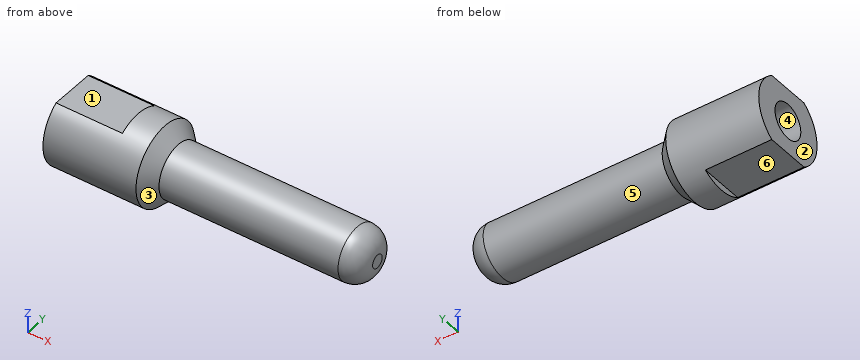
from build123d import *

# Parameters (mm, degrees)
F0_W        = 15.4432
F0_H        = 9.525
F3_DEPTH    = 15.875
F4_R        = 4.7752
F5_S5_R     = 6.35
F5_T6_DEPTH = 15
F7_D        = 8.4328
F7_DEPTH    = 19.685
F7_TIP      = 2.5334687141


# Not quite as in the source:
# - a fillet or chamfer that OpenCascade refuses, or shapes differently, is made with other operations: its cross-section is extruded or revolved along the edge and cut away or added


with BuildPart() as f1:
    # F0 (on Top) → F1 (revolve)
    with BuildSketch(Plane.XY):
        with Locations((-16.8899756006, 4.7625)):
            Rectangle(F0_W, F0_H)
        Polygon((-9.1683756006, 9.525), (-9.1683756006, 0), (48.4134243994, 0), (48.4134243994, 6.35), (0.8138243994, 6.35), (0.8138243994, 9.525), align=None)
    revolve(axis=Axis((11.9009243994, 0, 0), (1, 0, 0)))

    # F2 (on face) → F3 (cut)
    with BuildSketch(Plane(origin=(-24.6115756006, 0, 0), x_dir=(0, -1, 0), z_dir=(-1, 0, 0))):
        with BuildLine():
            ThreePointArc((5.2459455735, 7.9502), (0, 9.525), (-5.2459455735, 7.9502))
            Line((-5.2459455735, 7.9502), (5.2459455735, 7.9502))
        make_face()
        with BuildLine():
            Line((5.2651418547, -7.9375), (-5.2651418547, -7.9375))
            ThreePointArc((-5.2651418547, -7.9375), (0, -9.525), (5.2651418547, -7.9375))
        make_face()
    extrude(amount=-F3_DEPTH, mode=Mode.SUBTRACT)

    # F4
    f4_edges = [f1.edges().sort_by_distance(p)[0] for p in [
        (48.413424, -6.35, 0),
    ]]
    fillet(f4_edges, radius=F4_R)

    # F5: chamfer of 3.175 on 1 edges, made by hand


with BuildPart() as f5_tool2:
    # F5_s3 → F5_t4 (revolve)
    with BuildSketch(Plane.XY):
        Polygon((0.8138243994, 6.35), (-2.3611756006, 9.525), (0.8138243994, 9.525), align=None)
    revolve(axis=Axis((0.8138243994, 0, 0), (1, 0, 0)))

    # F5_s5 → F5_t6 (cut, symmetric)
    with BuildSketch(Plane.YZ.offset(-0.8)):
        Circle(F5_S5_R)
    extrude(amount=F5_T6_DEPTH, both=True, mode=Mode.SUBTRACT)


with BuildPart() as f1_1:
    add(f1.part)

    # F5_t1: cut F5_tool2
    add(f5_tool2.part, mode=Mode.SUBTRACT)

    # F7
    with Locations(Plane(origin=(-24.6115756006, 0, 0), x_dir=(0, -1, 0), z_dir=(-1, 0, 0))):
        with Locations((0, 0)):
            Hole(F7_D / 2, depth=F7_DEPTH)
            with Locations((0, 0, -(F7_DEPTH + F7_TIP / 2))):  # 118° drill point
                Cone(0, F7_D / 2, F7_TIP, mode=Mode.SUBTRACT)


solid = f1_1.part
Model file for the job. Use its own axes, mm. Face numbers are marked on the shaded views. A direction names the side the tool comes from. Round coordinates to 2 decimals unless told otherwise and drop trailing zeros. Loops run counter-clockwise (first coordinate to the right, second up) from the corner with the lowest first, then second, coordinate; pieces in that order, holes last. Notation, with made-up numbers: (8.25, 45.25) - (46.25, 45.25) arc R9 cw to (46.25, 54.25) - close; hole circle Ø9 at (27.5, 53.25). An arc over 180 degrees is marked (long way). Write each question's results on one line, items separated by ' | '.
(1) Pin check, flat tips, straight feed: pin 1 (4 mm diameter, centred on x = -8.5, z = -2.5, fed in from -Y); pin 2 (7.5 mm diameter, centred on y = 0, z = 0, fed in from -X); pin 3 (1.3 mm diameter, centred on y = 1.5, z = 8.5, fed in from -X); pin 4 (3 mm diameter, centred on x = -18.5, y = 1.5, fed in from -Z). Stop position of each tip, or through.
Answer below:
pin 1: stops at y = -9.51 | pin 2: stops at x = -4.65 | pin 3: stops at x = -24.61 | pin 4: stops at z = -7.94
(2) Mould opens along X. For the marked faces 1, 2 and 3 say: released by +X, released by -X, zero draft, split by the parting line, or undercut.
Answer below:
face 1: zero draft | face 2: released by -X | face 3: released by +X
(3) 3-axis set-ups, long thin cutter, end or side, ignore diameter. For the marked faces 4, 5 and 6: which of +Z, -Z, +X, -X, +Y, -Y reach the whole face in a straight line?
Answer below:
face 4: -X | face 5: +X | face 6: -Z, -X, +Y, -Y
(4) Saw through at A-A, the plane x = 33.5. List the corners of the cut face in (y, z), then the cut area to 3 significant figures.
Answer below:
outline: circle Ø12.7 at (0, 0) | area: 127 mm^2
(5) Wall check: L1, parallel to Z at x = -18.75, y = 0; L2, parallel to Y at x = -19.25, z = 0 (3 decimals); L3, parallel to Y at x = 21.5, z = 4.75. Give the ranges that are in metal, low to high.
Answer below:
L1: z = -7.94 to -4.22, 4.22 to 7.95 | L2: y = -9.525 to -4.216, 4.216 to 9.525 | L3: y = -4.21 to 4.21
